Input: part model. Units: mm. Frame: model coordinates. Round coordinates to 2 decimals unless told otherwise and drop trailing zeros. Write each loop counter-clockwise with the first axis right and the second up, starting at its lowest first coordinate (ties: lowest second). Pieces come first, ordered by that corner, then holes. Notation, with made-up numbers: (49, 36) -> (83, 36) arc R24 cw to (83, 52) -> close; hole circle Ø1 at (-15.75, 39.5). An arc over 180 degrees is marked (long way). Use CSV: the item, a comma, the result in double quotes.
```python
from build123d import *

# Parameters (mm, degrees)
F1_DEPTH = 19.05


with BuildPart() as f1:
    # F0 (on Front) → F1 (new body)
    with BuildSketch(Plane.XZ):
        with BuildLine():
            Line((47.313681, -11.632638), (314.013681, -11.632638))
            add(Edge.make_bspline(
                [(352.715969, 44.274099), (352.715969, 0), (335.928053, -9.905117), (314.013681, -11.632638)],
                knots=[0, 0, 0, 0, 67.995811, 67.995811, 67.995811, 67.995811], degree=3))
            add(Edge.make_bspline(
                [(284.34224, 50.548841), (313.035429, 139.851982), (348.589689, 97.368889), (352.715969, 44.274099)],
                knots=[0, 0, 0, 0, 68.661046, 68.661046, 68.661046, 68.661046], degree=3))
            Line((284.34224, 50.548841), (124.115969, 62.091228))
            add(Edge.make_bspline(
                [(79.665969, 63.324099), (102.446698, 82.186237), (124.115969, 68.843909), (124.115969, 62.091228)],
                knots=[0, 0, 0, 0, 44.467094, 44.467094, 44.467094, 44.467094], degree=3))
            add(Edge.make_bspline(
                [(-91.784031, 44.274099), (-69.512811, 66.651346), (-11.597474, 63.266684), (79.665969, 63.324099)],
                knots=[0, 0, 0, 0, 172.505087, 172.505087, 172.505087, 172.505087], degree=3))
            add(Edge.make_bspline(
                [(-91.784031, 44.274099), (-91.784031, 26.056429), (-69.163285, 21.455625), (-55.820961, 16.394742)],
                knots=[0, 0, 0, 0, 45.503857, 45.503857, 45.503857, 45.503857], degree=3))
            add(Edge.make_bspline(
                [(-55.820961, 16.394742), (-49.379837, 0), (-35.117339, -14.430643), (0, -11.632638)],
                knots=[0, 0, 0, 0, 62.462098, 62.462098, 62.462098, 62.462098], degree=3))
            add(Edge.make_bspline(
                [(47.313681, -11.632638), (39.288981, -19.225901), (10.748499, -19.225901), (0, -11.632638)],
                knots=[0, 0, 0, 0, 47.313681, 47.313681, 47.313681, 47.313681], degree=3))
        make_face()
    extrude(amount=F1_DEPTH)


solid = f1.part
```
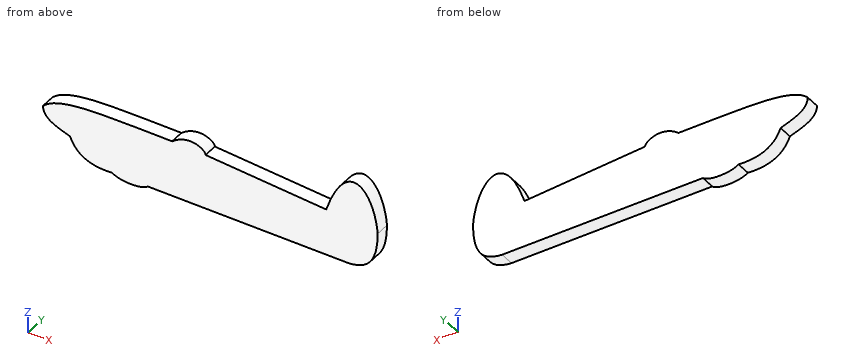
Item 1: First-contact query: pin 1 Ø10 at (x, y) = (289, -7.5) entering from -Z; pin 2 Ø8 at (x, y) = (-47, -5.5) entering from +Z; pin 3 Ø5 at (y, z) = (-4.5, 81.5) entering from +X. Flat tips, straight axial feed; report the tip coordinate or a pass-through.
Worked answers:
pin 1,"stops at z = -11.63"
pin 2,"stops at z = 61.22"
pin 3,"stops at x = 344.84"
Item 2: Section query A-A on x = 280.5. Return the cut outline in (y, z), plus the area to 3 significant figures.
Worked answers:
outline,"(-19.05, -11.63) -> (0, -11.63) -> (0, 50.83) -> (-19.05, 50.83) -> close"
area,"1,190 mm²"
Item 3: Line query: line 1 (Z direction, x = 50.5, y = -9.25); line 2 (Z direction, x = 8, y = -2.5); line 3 (X direction, y = -11, z = 67). Output: solid intervals per line, ascending.
Worked answers:
line 1,"z = -11.63 to 63.39"
line 2,"z = -15.2 to 63.42"
line 3,"x = 84.7 to 121.29, 290.29 to 348.88"
Item 4: Section query B-B on x = 149. Return the cut outline in (y, z).
Worked answers:
outline,"(-19.05, -11.63) -> (0, -11.63) -> (0, 60.3) -> (-19.05, 60.3) -> close"
